Build history of the part. All positions in model axes, mm. Face numbers are marked on the shaded views. Give positions to 0.01 mm unless a question says otherwise; leave off trailing zeros. Write each loop counter-clockwise with the first axis right and the second up, starting at its lowest first coordinate (ties: lowest second). Pieces come first, ordered by that corner, then holes. Notation, with made-up numbers: (-11, 78) -> (18, 78) arc R6 cw to (18, 87) -> close; hole circle Ø6 at (44.5, 42). An arc over 180 degrees is marked (long way). Put each result on its own line as item: value.
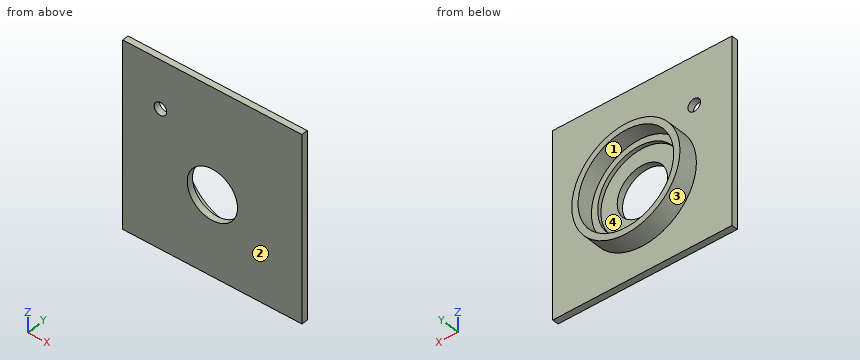
from build123d import *

# Parameters (mm, degrees)
F0_W      = 28.5
F0_H      = 29.5
F1_DEPTH  = 1
F3_R      = 4
F4_DEPTH  = 25
F5_R      = 8.6
F5_R_2    = 6.6
F6_DEPTH  = 0.6
F7_R      = 8.6
F7_R_2    = 7.6
F8_DEPTH  = 2.5
F9_R      = 1
F10_DEPTH = 25


with BuildPart() as f1:
    # F0 (on Front) → F1 (new body)
    with BuildSketch(Plane.XZ):
        with Locations((0, 2)):
            Rectangle(F0_W, F0_H)
    extrude(amount=F1_DEPTH)

    # F3 (on Front) → F4 (cut)
    with BuildSketch(Plane.XZ):
        Circle(F3_R)
    extrude(amount=F4_DEPTH, mode=Mode.SUBTRACT)

    # F5 (on face) → F6 (join)
    with BuildSketch(Plane(origin=(0, 0, 0), x_dir=(-1, 0, 0), z_dir=(0, 1, 0))):
        Circle(F5_R)
        Circle(F5_R_2, mode=Mode.SUBTRACT)
    extrude(amount=F6_DEPTH)

    # F7 (on face) → F8 (join)
    with BuildSketch(Plane(origin=(0, 0.6, 0), x_dir=(-1, 0, 0), z_dir=(0, 1, 0))):
        Circle(F7_R)
        Circle(F7_R_2, mode=Mode.SUBTRACT)
    extrude(amount=F8_DEPTH)

    # F9 (on face) → F10 (cut)
    with BuildSketch(Plane(origin=(0, 0, 0), x_dir=(-1, 0, 0), z_dir=(0, 1, 0))):
        with Locations((8.25, 9.1)):
            Circle(F9_R)
    extrude(amount=-F10_DEPTH, mode=Mode.SUBTRACT)


solid = f1.part
1) Slice it at B-B (x = 0). Write the cut outline in (y, z).
Filled sheet:
outline: (-1, -12.75) -> (0, -12.75) -> (0, -8.6) -> (3.1, -8.6) -> (3.1, -7.6) -> (0.6, -7.6) -> (0.6, -6.6) -> (0, -6.6) -> (0, -4) -> (-1, -4) -> close; (-1, 4) -> (0, 4) -> (0, 6.6) -> (0.6, 6.6) -> (0.6, 7.6) -> (3.1, 7.6) -> (3.1, 8.6) -> (0, 8.6) -> (0, 16.75) -> (-1, 16.75) -> close
2) Slice it at A-A (z = 9.1). Write the cut outline in (x, y).
Filled sheet:
outline: (-14.25, -1) -> (-9.25, -1) -> (-9.25, 0) -> (-14.25, 0) -> close; (-7.25, -1) -> (14.25, -1) -> (14.25, 0) -> (-7.25, 0) -> close
3) Slice it at D-D (z = 0). Write the cut outline in (x, y), plus the area to 3 significant figures.
Filled sheet:
outline: (-14.25, -1) -> (-4, -1) -> (-4, 0) -> (-6.6, 0) -> (-6.6, 0.6) -> (-7.6, 0.6) -> (-7.6, 3.1) -> (-8.6, 3.1) -> (-8.6, 0) -> (-14.25, 0) -> close; (4, -1) -> (14.25, -1) -> (14.25, 0) -> (8.6, 0) -> (8.6, 3.1) -> (7.6, 3.1) -> (7.6, 0.6) -> (6.6, 0.6) -> (6.6, 0) -> (4, 0) -> close
area: 27.9 mm2
4) Pin check, flat tips, straight feed: pin 1 (1.5 mm diameter, centred on x = -3, y = 1.5, fed in from +Z); pin 2 (4 mm diameter, centred on x = -10.5, z = -2, fed in from +Y); pin 3 (6.5 mm diameter, centred on x = 2.5, z = -2.5, fed in from +Y). Stop position of each tip, or through.
Filled sheet:
pin 1: z = 8.3
pin 2: y = 0
pin 3: y = 0.6
5) Wall check: L1, parallel to Z at x = 0, y = -0.35; L2, parallel to Z at x = -8.25, y = -0.6; L3, parallel to X at y = -0.05, z = 9. Give the ranges that are in metal, low to high.
Filled sheet:
L1: -12.75 to -4, 4 to 16.75
L2: -12.75 to 8.1, 10.1 to 16.75
L3: -14.25 to -9.24, -7.26 to 14.25
6) Pull direction Z, two halves, no side cores. Call the marked faces 1, 2, 3 and 4: released by +Z, released by -Z, zero draft, split by the parting line, or undercut.
Filled sheet:
face 1: undercut
face 2: zero draft
face 3: split by the parting line
face 4: undercut
7) Slice it at C-C (y = -0.4). Write the cut outline in (x, z), plus the area to 3 significant figures.
Filled sheet:
outline: (-14.25, -12.75) -> (14.25, -12.75) -> (14.25, 16.75) -> (-14.25, 16.75) -> close; hole circle Ø2 at (-8.25, 9.1); hole circle Ø8 at (0, 0)
area: 787 mm2
